Here's how the part is built. I have some questions about the finished solid (model axes, mm). A direction names the side the tool comes from. Round coordinates to 2 decimals unless told otherwise and drop trailing zeros. Order: outer loops, then holes, each group sorted by start corner. A loop starts at its lowest first (then second) coordinate and runs counter-clockwise, first axis right, second up.
```python
from build123d import *

# Parameters (mm, degrees)
BOSS_EXTRUDE1_DEPTH = 12.7
SKETCH2_W           = 330.2
SKETCH2_H           = 12.7
CUT_EXTRUDE1_DEPTH  = 6.35
CUT_EXTRUDE3_DEPTH  = 6.35


with BuildPart() as part:
    # Sketch1 → Boss-Extrude1 (new body)
    with BuildSketch(Plane.XY):
        Polygon((0, 0), (355.6, 0), (355.6, -223.774), (292.534512242, -286.839487758), (274.574, -304.8), (81.026, -304.8), (63.065487758, -286.839487758), (0, -223.774), align=None)
    extrude(amount=BOSS_EXTRUDE1_DEPTH)

    # Sketch2 → Cut-Extrude1 (cut)
    with BuildSketch(Plane.XY.offset(12.7)):
        Polygon((0, 0), (0, -223.774), (81.026, -304.8), (274.574, -304.8), (355.6, -223.774), (355.6, 0), align=None)
        Polygon((6.35, -221.143743879), (67.607470696, -282.401214575), (64.787670274, -285.221014997), (82.004455277, -302.4378), (83.656256121, -298.45), (271.943743879, -298.45), (273.595544723, -302.4378), (290.812329726, -285.221014997), (287.992529304, -282.401214575), (349.25, -221.143743879), (349.25, -6.35), (6.35, -6.35), align=None, mode=Mode.SUBTRACT)
        with Locations((177.8, -44.45)):
            Rectangle(SKETCH2_W, SKETCH2_H)
    extrude(amount=-CUT_EXTRUDE1_DEPTH, mode=Mode.SUBTRACT)

    # Sketch3 → Cut-Extrude3 (cut)
    with BuildSketch(Plane.XY.offset(12.7)):
        Polygon((85.308056965, -294.4622), (70.400831804, -279.554974839), (74.890959865, -275.064846778), (87.938313086, -288.1122), align=None)
        Polygon((285.199168196, -279.554974839), (280.709040135, -275.064846778), (267.661686914, -288.1122), (270.291943035, -294.4622), align=None)
    extrude(amount=-CUT_EXTRUDE3_DEPTH, mode=Mode.SUBTRACT)


solid = part.part
```
1) If we section it at C-C (y = -216): Write out the boundary of the cut face in (x, z).
2) If we section it at D-D (y = -258): Write out the boundary of the cut face in (x, z).
3) I need wall thicknesses on line 1 (Y direction, x = 170, z = 10.75); line 2 (Z direction, x = 160.5, y = -39); line 3 (X direction, y = -60, z = 11). Which ranges of each line are inside material? Lowest first, please.
4) If we section it at B-B (x = 203): Write out the boundary of the cut face in (y, z).
5) I'm going to push flat-ended pins straight in: pin 1 (3 mm diameter, centred on y = -91, z = 8, fed in from +X); pin 2 (1.9 mm diameter, centred on x = 224.5, z = 8.5, fed in from +Y); pin 3 (3 mm diameter, centred on y = -47, z = 11, fed in from -X). Where does each tip first touch, or does it pass through?
6) If we section it at A-A (z = 9.25): Write out the boundary of the cut face in (x, y).
7) We'd pull the mould along X, two halves only. Please class faces 1 (the flat face through (318.192, -252.201, 9.569)), 2 (the flat face through (274.277, -281.497, 9.569)), 3 (the flat face through (73.276, -293.709, 9.569)): +X half, -X half, draft (parallel to the pull), parting line (faces both ways), or undercut.
8) For faces 4 (the flat face through (180, -150, 0)), 5 (the flat face through (282.083, -293.95, 9.569)), 6 (the flat face through (175, -44, 6.35)), which set-ups out of +Z, -Z, +X, -X, +Y, -Y let a thin tool reach every point of the face, with its end or its side?
Solutions:
1. outline: (0, 0) - (355.6, 0) - (355.6, 6.35) - (349.25, 6.35) - (349.25, 12.7) - (6.35, 12.7) - (6.35, 6.35) - (0, 6.35) - close
2. outline: (34.23, 0) - (321.37, 0) - (321.37, 6.35) - (312.39, 6.35) - (312.39, 12.7) - (43.21, 12.7) - (43.21, 6.35) - (34.23, 6.35) - close
3. line 1: y = -298.45 to -50.8, -38.1 to -6.35
3. line 2: z = 0 to 6.35
3. line 3: x = 6.35 to 349.25
4. outline: (-304.8, 0) - (0, 0) - (0, 6.35) - (-6.35, 6.35) - (-6.35, 12.7) - (-38.1, 12.7) - (-38.1, 6.35) - (-50.8, 6.35) - (-50.8, 12.7) - (-298.45, 12.7) - (-298.45, 6.35) - (-304.8, 6.35) - close
5. pin 1: stops at x = 349.25
5. pin 2: stops at y = -6.35
5. pin 3: stops at x = 6.35
6. outline: (6.35, -221.14) - (67.61, -282.4) - (64.79, -285.22) - (82, -302.44) - (83.66, -298.45) - (271.94, -298.45) - (273.6, -302.44) - (290.81, -285.22) - (287.99, -282.4) - (349.25, -221.14) - (349.25, -6.35) - (6.35, -6.35) - close; hole (12.7, -50.8) - (342.9, -50.8) - (342.9, -38.1) - (12.7, -38.1) - close; hole (70.4, -279.55) - (85.31, -294.46) - (87.94, -288.11) - (74.89, -275.06) - close; hole (267.66, -288.11) - (270.29, -294.46) - (285.2, -279.55) - (280.71, -275.06) - close
7. face 1: +X half
7. face 2: undercut
7. face 3: -X half
8. face 4: -Z, +X, -X, +Y, -Y
8. face 5: +Z, +X, -Y
8. face 6: +Z
